Autodesk Inventor part; units mm, degrees
ref_plane "YZ Plane" through (0, 0, 0) normal (1, 0, 0) x (0, 1, 0)
ref_plane "XZ Plane" through (0, 0, 0) normal (0, 1, 0) x (-1, 0, 0)
ref_plane "XY Plane" through (0, 0, 0) normal (0, 0, 1) x (1, 0, 0)
sketch "Sketch1" plane through (0, 0, 0) normal (0, 0, 1) x (1, 0, 0)
  line L0 (-44, -7.75) -> (44, -7.75)
  line L1 (44, -7.75) -> (44, 7.75)
  line L2 (44, 7.75) -> (-44, 7.75)
  line L3 (-44, 7.75) -> (-44, -7.75)
  line L4 (-44, -7.75) -> (44, 7.75) construction
  line L5 (44, -7.75) -> (-44, 7.75) construction
  line L6 (-44, -7.75) -> (44, -7.75)
  line L7 (44, -7.75) -> (44, -11.75)
  line L8 (44, -11.75) -> (-44, -11.75)
  line L9 (-44, -11.75) -> (-44, -7.75)
  line L10 (-44, 7.75) -> (-21, 7.75)
  line L11 (-21, 7.75) -> (-21, 11.75)
  line L12 (-21, 11.75) -> (-44, 11.75)
  line L13 (-44, 11.75) -> (-44, 7.75)
  line L14 (44, 7.75) -> (21, 7.75)
  line L15 (21, 7.75) -> (21, 11.75)
  line L16 (21, 11.75) -> (44, 11.75)
  line L17 (44, 11.75) -> (44, 7.75)
  line L18 (0, 0) -> (0, -41.0889) construction
  circle A0 centre (0, -21) radius 9.25
  circle A1 centre (0, -21) radius 13.25
  line L19 (-13.25, -21) -> (-13.25, -11.75)
  line L20 (-13.25, -11.75) -> (-9.4868, -11.75)
  line L21 (13.25, -11.75) -> (9.4868, -11.75)
  line L22 (13.25, -21) -> (13.25, -11.75)
  line L23 (13.25, -11.75) -> (9.4868, -11.75)
  line L24 (0, 0) -> (65.293, 0) construction
  line L25 (21, -7.75) -> (6, -7.75)
  line L26 (6, -7.75) -> (6, 7.75)
  line L27 (6, 7.75) -> (21, 7.75)
  line L28 (21, 7.75) -> (21, -7.75)
  line L29 (21, -7.75) -> (6, 7.75) construction
  line L30 (6, -7.75) -> (21, 7.75) construction
  point P0 (13.25, -21)
  point P1 (13.5, 0)
  dimension "d0" = 88
  dimension "d1" = 15.5
  dimension "d2" = 4
  dimension "d3" = 4
  dimension "d4" = 23
  dimension "d5" = 23
  dimension "d6" = 18.5
  dimension "d7" = 26.5
  dimension "d8" = 90
  dimension "d19" = 15
  dimension "d20" = 15.5
  dimension "d21" = 23
extrude "main" add sketch "Sketch1" along normal blind 32 contours L0 L7 L8 A1 | A1 L8 L9 L0 | A1 L8 | L15 L16 L17 L2 | A1 L8 | L8 L22 A1 | A1 L19 L8 | L2 L13 L12 L11
extrude "bottom" add sketch "Sketch1" along normal blind 4 contours L0 L3 L2 L26 | L28 L2 L1 L0
fillet "Fillet1" radius 15 2 edges at (13.25, -11.75, 16) (-13.25, -11.75, 16)
fillet "Fillet2" radius 4 8 edges at (-44, 11.75, 16) (-44, -11.75, 16) (44, 11.75, 16) (44, -11.75, 16) (32.5, 11.75, 32) (-32.5, 11.75, 32) (21, -7.75, 2) (6, -7.75, 2)
equation "\"d2\" = wall"
equation "\"d3\" = wall2"
equation "\"d4\" = d5"
equation "\"d5\" = d21"
equation "\"d7\" = d6 + 2 * wall"
equation "\"d20\" = d1"
equation "\"d15\" = wall"
equation "\"d14\" = wall"
equation "\"wall\" = 4"
equation "\"wall2\" = 4"
properties part number "camera_holder"
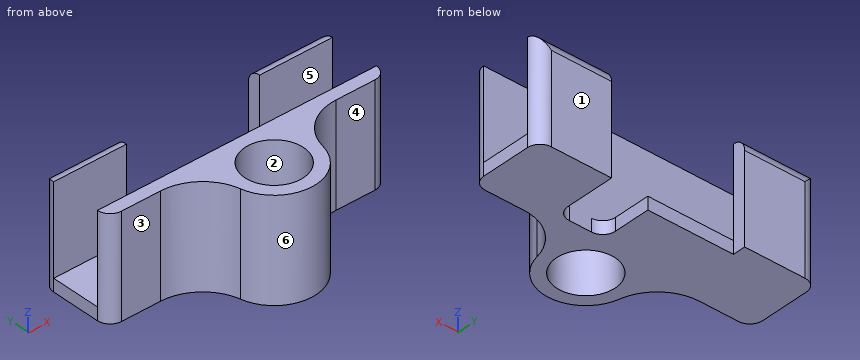
Work out the finished part from the listing and answer in its coordinate system (mm). Face numbers are marked on the shaded views. A direction names the side the tool comes from. Coordinates: 2 decimals unless noted, no trailing zeros. Loops run counter-clockwise (first coordinate to the right, second up) from the corner with the lowest first, then second, coordinate; pieces in that order, holes last. Notation, with made-up numbers: (44, 70.25) -> (100, 70.25) arc R16 ccw to (100, 76.25) -> close; hole circle Ø9 at (40.25, 58). An arc over 180 degrees is marked (long way). Answer as CSV lines item,"result".
1) The part is cut by section C-C (z = 11.5). State how many separate pieces and enclosed holes the cut face has, and give its area (3 significant figures).
A:
separate pieces,"3"
enclosed holes,"1"
area,"857 mm²"
2) For the marked faces 4, 5 and 6, determine the directions among +Z, -Z, +X, -X, +Y, -Y from which every point of the face is accessible in a straight line to the end or side of a thin tool.
A:
face 4,"+Z, -Z, +X, -Y"
face 5,"+Z, +X, -X"
face 6,"+Z, -Z, -Y"
3) The part is cut by section A-A (y = 1). Give the vertices of the cut face in (x, z), and give its area (3 significant figures).
A:
outline,"(-44, 0) -> (6, 0) -> (6, 4) -> (-44, 4) -> close; (21, 0) -> (44, 0) -> (44, 4) -> (21, 4) -> close"
area,"292 mm²"
4) Flat-ended cylindrical pins translate along their axes: pin 1 (12 mm diameter, centred on x = -30.5, z = 23.5, fed in from -Y); pin 2 (12 mm diameter, centred on x = -27.5, y = -18.5, fed in from -Z); pin 3 (12 mm diameter, centred on x = 13, z = 11.5, fed in from -Y); pin 4 (8 mm diameter, centred on x = 12.5, z = 7.5, fed in from +Y). Find the tip coordinate at first contact, or state that the pin passes through.
A:
pin 1,"stops at y = -12.09"
pin 2,"passes through"
pin 3,"stops at y = -32.25"
pin 4,"stops at y = -7.75"
5) The part is cut by section B-B (x = 0). Give the vertices of the cut face in (y, z).
A:
outline,"(-34.25, 0) -> (-30.25, 0) -> (-30.25, 32) -> (-34.25, 32) -> close; (-11.75, 0) -> (7.75, 0) -> (7.75, 4) -> (-7.75, 4) -> (-7.75, 32) -> (-11.75, 32) -> close"
6) For a pull along Y with two mould halves and no side action, classify the marked faces 1, 2 and 3 as released by +Y, released by -Y, zero draft, split by the parting line, or undercut.
A:
face 1,"released by +Y"
face 2,"undercut"
face 3,"released by -Y"
7) Straight lines are drawn through the part: probe 1 along Y at (x, z) = (39, 7.5); probe 2 along Z at (x, y) = (-4.5, -4.5); probe 3 along Y at (x, z) = (25.5, 10). For each, find the intervals that lie inside material, in ascending order.
A:
probe 1,"y = -11.75 to -7.75, 7.75 to 11.75"
probe 2,"z = 0 to 4"
probe 3,"y = -11.91 to -7.75, 7.75 to 11.75"
